from build123d import *

# Parameters (mm, degrees)
SKETCH1_W           = 101.6
SKETCH1_H           = 50.8
BOSS_EXTRUDE1_DEPTH = 7.5
SKETCH2_W           = 94.25
SKETCH2_H           = 43.45
BOSS_EXTRUDE2_DEPTH = 7.5
SKETCH3_R           = 2.75
CUT_EXTRUDE1_DEPTH  = 59.74351028
FILLET1_R           = 6
SKETCH4_R           = 3
SKETCH4_R_2         = 2.5
CUT_EXTRUDE2_DEPTH  = 7.5
CHAMFER1_SIZE       = 2
CHAMFER2_SIZE       = 3


with BuildPart() as part:
    # Sketch1 → Boss-Extrude1 (new body)
    with BuildSketch(Plane.XY):
        Rectangle(SKETCH1_W, SKETCH1_H)
    extrude(amount=-BOSS_EXTRUDE1_DEPTH)

    # Sketch2 → Boss-Extrude2 (add)
    with BuildSketch(Plane(origin=(0, 0, -7.5), x_dir=(-1, 0, 0), z_dir=(0, 0, -1))):
        Rectangle(SKETCH2_W, SKETCH2_H)
    extrude(amount=BOSS_EXTRUDE2_DEPTH)

    # Sketch3 → Cut-Extrude1 (cut, through all)
    with BuildSketch(Plane.XY):
        with Locations((-19, 0)):
            Circle(SKETCH3_R)
        with Locations((-13.435028843, 13.435028843)):
            Circle(SKETCH3_R)
        with Locations((13.435028843, 13.435028843)):
            Circle(SKETCH3_R)
        with Locations((19, 0)):
            Circle(SKETCH3_R)
        with Locations((13.435028843, -13.435028843)):
            Circle(SKETCH3_R)
        with Locations((-13.435028843, -13.435028843)):
            Circle(SKETCH3_R)
        with BuildLine():
            Line((8.5, 5.547296639), (8.5, 25.4))
            Line((8.5, 25.4), (-8.5, 25.4))
            Line((-8.5, 25.4), (-8.5, 5.547296639))
            ThreePointArc((-8.5, 5.547296639), (0, -10.15), (8.5, 5.547296639))
        make_face()
    extrude(amount=-CUT_EXTRUDE1_DEPTH, mode=Mode.SUBTRACT)

    # Fillet1
    fillet1_edges = [part.edges().sort_by_distance(p)[0] for p in [
        (-50.8, 25.4, -3.75),
        (50.8, 25.4, -3.75),
        (50.8, -25.4, -3.75),
        (-50.8, -25.4, -3.75),
    ]]
    fillet(fillet1_edges, radius=FILLET1_R)

    # Sketch4 → Cut-Extrude2 (cut)
    with BuildSketch(Plane(origin=(0, 0, -15), x_dir=(-1, 0, 0), z_dir=(0, 0, -1))):
        with Locations((-47.125, 21.725)):
            Circle(SKETCH4_R)
        with Locations((-47.125, -21.725)):
            Circle(SKETCH4_R)
        with Locations((-47.125, 0)):
            Circle(SKETCH4_R_2)
        with Locations((0, -21.725)):
            Circle(SKETCH4_R_2)
        with Locations((47.125, -21.725)):
            Circle(SKETCH4_R)
        with Locations((47.125, 0)):
            Circle(SKETCH4_R_2)
        with Locations((47.125, 21.725)):
            Circle(SKETCH4_R)
    extrude(amount=-CUT_EXTRUDE2_DEPTH, mode=Mode.SUBTRACT)

    # Chamfer1
    chamfer1_edges = [part.edges().sort_by_distance(p)[0] for p in [
        (-26.65, 25.4, 0),
        (0, -25.4, 0),
        (-50.8, 0, 0),
        (50.8, 0, 0),
        (26.65, 25.4, 0),
        (49.042640687, 23.642640687, 0),
        (-49.042640687, 23.642640687, 0),
        (-49.042640687, -23.642640687, 0),
        (49.042640687, -23.642640687, 0),
    ]]
    chamfer(chamfer1_edges, length=CHAMFER1_SIZE)

    # Chamfer2
    # the kernel refuses this chamfer: 3 mm, written as the material it takes off along each edge
    with BuildSketch(Plane(origin=(-13.435028843, -13.435028843, -15), x_dir=(1, 0, 0), z_dir=(0, -1, 0))) as chamfer2_piece_1:
        Polygon((2.75, CHAMFER2_SIZE), (2.75 + CHAMFER2_SIZE, 0), (2.75, 0), align=None)
    revolve(axis=Axis((-13.435028843, -13.435028843, -15), (0, 0, 1)), mode=Mode.SUBTRACT)
    with BuildSketch(Plane(origin=(13.435028843, -13.435028843, -15), x_dir=(1, 0, 0), z_dir=(0, -1, 0))) as chamfer2_piece_2:
        Polygon((2.75, CHAMFER2_SIZE), (2.75 + CHAMFER2_SIZE, 0), (2.75, 0), align=None)
    revolve(axis=Axis((13.435028843, -13.435028843, -15), (0, 0, 1)), mode=Mode.SUBTRACT)
    with BuildSketch(Plane(origin=(19, 0, -15), x_dir=(1, 0, 0), z_dir=(0, -1, 0))) as chamfer2_piece_3:
        Polygon((2.75, CHAMFER2_SIZE), (2.75 + CHAMFER2_SIZE, 0), (2.75, 0), align=None)
    revolve(axis=Axis((19, 0, -15), (0, 0, 1)), mode=Mode.SUBTRACT)
    with BuildSketch(Plane(origin=(13.435028843, 13.435028843, -15), x_dir=(1, 0, 0), z_dir=(0, -1, 0))) as chamfer2_piece_4:
        Polygon((2.75, CHAMFER2_SIZE), (2.75 + CHAMFER2_SIZE, 0), (2.75, 0), align=None)
    revolve(axis=Axis((13.435028843, 13.435028843, -15), (0, 0, 1)), mode=Mode.SUBTRACT)
    with BuildSketch(Plane(origin=(-13.435028843, 13.435028843, -15), x_dir=(1, 0, 0), z_dir=(0, -1, 0))) as chamfer2_piece_5:
        Polygon((2.75, CHAMFER2_SIZE), (2.75 + CHAMFER2_SIZE, 0), (2.75, 0), align=None)
    revolve(axis=Axis((-13.435028843, 13.435028843, -15), (0, 0, 1)), mode=Mode.SUBTRACT)
    with BuildSketch(Plane(origin=(-19, 0, -15), x_dir=(1, 0, 0), z_dir=(0, -1, 0))) as chamfer2_piece_6:
        Polygon((2.75, CHAMFER2_SIZE), (2.75 + CHAMFER2_SIZE, 0), (2.75, 0), align=None)
    revolve(axis=Axis((-19, 0, -15), (0, 0, 1)), mode=Mode.SUBTRACT)


solid = part.part
CAD build for the part. Positions are in the model's coordinates, mm. A direction names the side the tool comes from. Round coordinates to 2 decimals unless told otherwise and drop trailing zeros. Loops run counter-clockwise (first coordinate to the right, second up) from the corner with the lowest first, then second, coordinate; pieces in that order, holes last.
(1) Which spindle directions (+Z, -Z, +X, -X, +Y, -Y) get a long thin tool onto all of the face, cutting with end or side? Do faces 1 (the cylindrical face through (44.98, -19.63, -11.3)), 2 (the flat face through (27, 21.725, -11)), 3 (the cylindrical face through (45.03, 19.58, -11.3)), 4 (the cylindrical face through (44.626, -0.055, -11.302)), 5 (the flat face through (8.5, 15, -7)). Say none if no direction does.
(2) Cut at B-B (x = -42). Give the cut face in (y, z) (3 decimals).
(3) Cut at C-C (z = -13). Give the cut face in (x, y) (3 decimals).
(4) Drop flat-ended pins along their axis: pin 1 (8 mm diameter, centred on y = -13, z = -13, fed in from -X) (3 decimals); pin 2 (7 mm diameter, centred on x = 13.44, y = 13.44, fed in from -Z); pin 3 (8 mm diameter, centred on y = -7, z = -12, fed in from +X) (3 decimals). Give the stop position or say it passes through.
(5) Wall check: line 1 along X through (y, z) = (-14, -8) (3 decimals); line 2 along X through (y, z) = (-12, -12.25) (1 decimal); line 3 along X through (y, z) = (2, -13.75) (3 decimals). Give the ranges that are in metal, low to high.
(6) Cut at A-A (y = 0). Give the cut face in (x, z) (3 decimals).
(7) Two-plate mould, pull along Y, no slides. Class faces 6 (the flat face through (-1, -25.4, -5)), 7 (the conical face through (48.131, 22.805, -0.764)), 8 (the cylindrical face through (11.408, 15.294, -5.916)): +Y half, -Y half, draft (parallel to the pull), parting line (faces both ways), or undercut.
(8) Cut at D-D (x = 15). State how many separate pieces and enclosed holes the cut face has, plus the area to 3 significant figures.
Findings below:
1. face 1: -Z, +X, -Y
1. face 2: -Z, +X, -X, +Y
1. face 3: -Z, +X, +Y
1. face 4: -Z, +X
1. face 5: +Z, -Z, +Y
2. outline: (-25.4, -7.5) - (-21.725, -7.5) - (-21.725, -15) - (21.725, -15) - (21.725, -7.5) - (25.4, -7.5) - (25.4, -2) - (23.4, 0) - (-23.4, 0) - (-25.4, -2) - close
3. outline: (-47.125, -18.725) arc R3 cw to (-44.125, -21.725) - (-2.5, -21.725) arc R2.5 cw to (2.5, -21.725) - (44.125, -21.725) arc R3 cw to (47.125, -18.725) - (47.125, -2.5) arc R2.5 cw to (47.125, 2.5) - (47.125, 18.725) arc R3 cw to (44.125, 21.725) - (8.5, 21.725) - (8.5, 5.547) arc R10.15 cw (long way) to (-8.5, 5.547) - (-8.5, 21.725) - (-44.125, 21.725) arc R3 cw to (-47.125, 18.725) - (-47.125, 2.5) arc R2.5 cw to (-47.125, -2.5) - close; hole circle Ø7.5 at (-19, 0); hole circle Ø7.5 at (-13.435, -13.435); hole circle Ø7.5 at (-13.435, 13.435); hole circle Ø7.5 at (13.435, -13.435); hole circle Ø7.5 at (13.435, 13.435); hole circle Ø7.5 at (19, 0)
4. pin 1: stops at x = -47.125
4. pin 2: stops at z = -12.76
4. pin 3: stops at x = 47.125
5. line 1: x = -47.125 to -16.126, -10.744 to 10.744, 16.126 to 47.125
5. line 2: x = -47.1 to -16.1, -10.8 to 10.8, 16.1 to 47.1
5. line 3: x = -45.625 to -23.031, -14.969 to -9.951, 9.951 to 14.969, 23.031 to 45.625
6. outline: (-50.8, -7.5) - (-44.625, -7.5) - (-44.625, -15) - (-24.75, -15) - (-21.75, -12) - (-21.75, 0) - (-48.8, 0) - (-50.8, -2) - close; (-16.25, -12) - (-13.25, -15) - (-10.15, -15) - (-10.15, 0) - (-16.25, 0) - close; (10.15, -15) - (13.25, -15) - (16.25, -12) - (16.25, 0) - (10.15, 0) - close; (21.75, -12) - (24.75, -15) - (44.625, -15) - (44.625, -7.5) - (50.8, -7.5) - (50.8, -2) - (48.8, 0) - (21.75, 0) - close
7. face 6: -Y half
7. face 7: +Y half
7. face 8: undercut
8. separate pieces: 3
8. enclosed holes: 0
8. area: 538 mm2
